CAD build for the part. Positions are in the model's coordinates, mm. Round coordinates to 2 decimals unless told otherwise and drop trailing zeros. Answer as a JSON object with one key per item and string values. Group by question number.
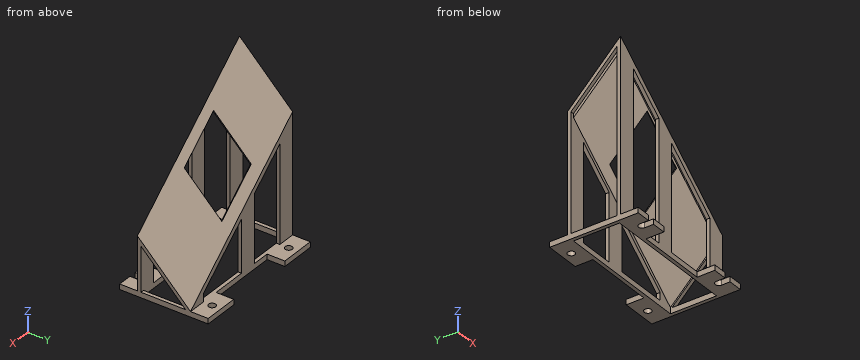
```python
from build123d import *

# Parameters (mm, degrees)
SKETCH_2_W           = 240
SKETCH_2_H           = 150
EXTRUDE_1_DEPTH      = 250
CUT_EXTRUDE_1_DEPTH  = 200
CUT_REVOLVE_1_ANGLE  = 37.4
SKETCH_13_W          = 80
SKETCH_13_H          = 100
CUT_EXTRUDE_2_DEPTH  = 295
SKETCH_14_W          = 160
SKETCH_14_H          = 150
CUT_EXTRUDE_3_DEPTH  = 295
SKETCH_16_W          = 80
SKETCH_16_H          = 28.16
CUT_EXTRUDE_4_DEPTH  = 295
SKETCH_22_W          = 80
SKETCH_22_H          = 9.999058643
CUT_EXTRUDE_5_DEPTH  = 120
SKETCH_23_W          = 80
SKETCH_23_H          = 9.99833939
CUT_EXTRUDE_6_DEPTH  = 142
SKETCH_24_W          = 80
SKETCH_24_H          = 11.98
CUT_EXTRUDE_7_DEPTH  = 142
SKETCH_25_W          = 20
SKETCH_25_H          = 3
EXTRUDE_2_DEPTH      = 10
SKETCH_26_W          = 20
SKETCH_26_H          = 3
EXTRUDE_3_DEPTH      = 10
SKETCH_27_W          = 20
SKETCH_27_H          = 3
EXTRUDE_4_DEPTH      = 10
SKETCH_28_W          = 20
SKETCH_28_H          = 3
EXTRUDE_5_DEPTH      = 10
SKETCH_29_R          = 1.997024656
CUT_EXTRUDE_8_DEPTH  = 10
SKETCH_30_R          = 1.996157305
CUT_EXTRUDE_9_DEPTH  = 10
CUT_EXTRUDE_10_DEPTH = 10
CUT_EXTRUDE_11_DEPTH = 10
SKETCH_34_W          = 76
SKETCH_34_H          = 26.002601967
CUT_EXTRUDE_14_DEPTH = 2
CUT_EXTRUDE_15_DEPTH = 2
CUT_EXTRUDE_17_DEPTH = 2
CUT_EXTRUDE_18_DEPTH = 2
CUT_EXTRUDE_20_DEPTH = 2
CUT_EXTRUDE_22_DEPTH = 2


with BuildPart() as part:
    # 草图2 → 凸台-拉伸1 (new body)
    with BuildSketch(Plane.XY):
        Rectangle(SKETCH_2_W, SKETCH_2_H)
    extrude(amount=EXTRUDE_1_DEPTH)

    # 草图9 → 切除-拉伸1 (cut)
    with BuildSketch(Plane(origin=(0, 75, 0), x_dir=(1, 0, 0), z_dir=(0, 1, 0))):
        Polygon((120, -250), (-120, -250), (208.236072982, 25.422767778), align=None)
    extrude(amount=-CUT_EXTRUDE_1_DEPTH, mode=Mode.SUBTRACT)

    # 草图10 → 切除-旋转1 (revolve, cut)
    with BuildSketch(Plane(origin=(73.519859787, 0, 87.617557028), x_dir=(0.7660444431189816, 0, -0.6427876096865353), z_dir=(0.6427876096865353, 0, 0.7660444431189817))):
        Polygon((60.675513844, -75), (-252.622235596, -75), (-252.622235596, 287.743692907), (60.675513844, 234.486341656), align=None)
    revolve(axis=Axis((120, -75, 48.616088517), (-0.7660444431189815, 0, 0.6427876096865353)), revolution_arc=CUT_REVOLVE_1_ANGLE, mode=Mode.SUBTRACT)

    # 草图13 → 切除-拉伸2 (cut)
    with BuildSketch(Plane(origin=(0, 0, 0), x_dir=(-1, 0, 0), z_dir=(0, 0, -1))):
        with Locations((80, -25)):
            Rectangle(SKETCH_13_W, SKETCH_13_H)
    extrude(amount=-CUT_EXTRUDE_2_DEPTH, mode=Mode.SUBTRACT)

    # 草图14 → 切除-拉伸3 (cut)
    with BuildSketch(Plane(origin=(0, 0, 0), x_dir=(-1, 0, 0), z_dir=(0, 0, -1))):
        with Locations((-40, 0)):
            Rectangle(SKETCH_14_W, SKETCH_14_H)
    extrude(amount=-CUT_EXTRUDE_3_DEPTH, mode=Mode.SUBTRACT)

    # 草图16 → 切除-拉伸4 (cut)
    with BuildSketch(Plane(origin=(0, 75, 0), x_dir=(1, 0, 0), z_dir=(0, 1, 0))):
        with Locations((-80, -14.08)):
            Rectangle(SKETCH_16_W, SKETCH_16_H)
    extrude(amount=-CUT_EXTRUDE_4_DEPTH, mode=Mode.SUBTRACT)

    # 草图22 → 切除-拉伸5 (cut)
    with BuildSketch(Plane(origin=(0, 0, 28.16), x_dir=(-1, 0, 0), z_dir=(0, 0, -1))):
        with Locations((80, 70.000470678)):
            Rectangle(SKETCH_22_W, SKETCH_22_H)
    extrude(amount=-CUT_EXTRUDE_5_DEPTH, mode=Mode.SUBTRACT)

    # 草图23 → 切除-拉伸6 (cut)
    with BuildSketch(Plane(origin=(0, 0, 28.16), x_dir=(-1, 0, 0), z_dir=(0, 0, -1))):
        with Locations((80, 29.999169695)):
            Rectangle(SKETCH_23_W, SKETCH_23_H)
    extrude(amount=-CUT_EXTRUDE_6_DEPTH, mode=Mode.SUBTRACT)

    # 草图24 → 切除-拉伸7 (cut)
    with BuildSketch(Plane(origin=(0, 65.000941357, 0), x_dir=(1, 0, 0), z_dir=(0, 1, 0))):
        with Locations((-80, -34.15)):
            Rectangle(SKETCH_24_W, SKETCH_24_H)
    extrude(amount=-CUT_EXTRUDE_7_DEPTH, mode=Mode.SUBTRACT)

    # 草图25 → 凸台-拉伸2 (add)
    with BuildSketch(Plane(origin=(0, 65.000941357, 0), x_dir=(1, 0, 0), z_dir=(0, 1, 0))):
        with Locations((-50, -41.64)):
            Rectangle(SKETCH_25_W, SKETCH_25_H)
    extrude(amount=EXTRUDE_2_DEPTH)

    # 草图26 → 凸台-拉伸3 (add)
    with BuildSketch(Plane(origin=(0, 65.000941357, 0), x_dir=(1, 0, 0), z_dir=(0, 1, 0))):
        with Locations((-110, -41.64)):
            Rectangle(SKETCH_26_W, SKETCH_26_H)
    extrude(amount=EXTRUDE_3_DEPTH)

    # 草图27 → 凸台-拉伸4 (add)
    with BuildSketch(Plane.XZ.offset(-34.99833939)):
        with Locations((-50, 41.64)):
            Rectangle(SKETCH_27_W, SKETCH_27_H)
    extrude(amount=EXTRUDE_4_DEPTH)

    # 草图28 → 凸台-拉伸5 (add)
    with BuildSketch(Plane.XZ.offset(-34.99833939)):
        with Locations((-110, 41.64)):
            Rectangle(SKETCH_28_W, SKETCH_28_H)
    extrude(amount=EXTRUDE_5_DEPTH)

    # 草图29 → 切除-拉伸8 (cut)
    with BuildSketch(Plane.XY.offset(43.14)):
        with Locations((-110, 69.998446832)):
            Circle(SKETCH_29_R)
    extrude(amount=-CUT_EXTRUDE_8_DEPTH, mode=Mode.SUBTRACT)

    # 草图30 → 切除-拉伸9 (cut)
    with BuildSketch(Plane.XY.offset(43.14)):
        with Locations((-50, 70.000941357)):
            Circle(SKETCH_30_R)
    extrude(amount=-CUT_EXTRUDE_9_DEPTH, mode=Mode.SUBTRACT)

    # 草图31 → 切除-拉伸10 (cut)
    with BuildSketch(Plane(origin=(0, 0, 40.14), x_dir=(-1, 0, 0), z_dir=(0, 0, -1))):
        with BuildLine():
            ThreePointArc((52, 29.962991919), (50, 31.962991919), (48, 29.962991919))
            Line((48, 29.962991919), (50, 29.962991919))
            Line((50, 29.962991919), (52, 29.962991919))
        make_face()
        with BuildLine():
            Line((48, 29.962991919), (48, 24.99833939))
            Line((48, 24.99833939), (50, 24.99833939))
            Line((50, 24.99833939), (50, 27.962991919))
            ThreePointArc((50, 27.962991919), (48.585786438, 28.548778357), (48, 29.962991919))
        make_face()
        with BuildLine():
            Line((50, 27.962991919), (50, 24.99833939))
            Line((50, 24.99833939), (52, 24.99833939))
            Line((52, 24.99833939), (52, 29.962991919))
            ThreePointArc((52, 29.962991919), (51.414213562, 28.548778357), (50, 27.962991919))
        make_face()
        with BuildLine():
            Line((50, 29.962991919), (48, 29.962991919))
            ThreePointArc((48, 29.962991919), (48.585786438, 28.548778357), (50, 27.962991919))
            Line((50, 27.962991919), (50, 29.962991919))
        make_face()
        with BuildLine():
            Line((50, 29.962991919), (50, 27.962991919))
            ThreePointArc((50, 27.962991919), (51.414213562, 28.548778357), (52, 29.962991919))
            Line((52, 29.962991919), (50, 29.962991919))
        make_face()
    extrude(amount=-CUT_EXTRUDE_10_DEPTH, mode=Mode.SUBTRACT)

    # 草图32 → 切除-拉伸11 (cut)
    with BuildSketch(Plane(origin=(0, 0, 40.14), x_dir=(-1, 0, 0), z_dir=(0, 0, -1))):
        with BuildLine():
            Line((112, 24.99833939), (112, 29.99833939))
            ThreePointArc((112, 29.99833939), (110, 31.99833939), (108, 29.99833939))
            Line((108, 29.99833939), (108, 24.99833939))
            Line((108, 24.99833939), (112, 24.99833939))
        make_face()
    extrude(amount=-CUT_EXTRUDE_11_DEPTH, mode=Mode.SUBTRACT)

    # 抽壳9: read off the stored shape, not the designer's step
    # 抽壳9: loft between two sections, ruled curve by curve
    shell_9_from = [
        Edge.make_line((-118, 36.99833939, 133.254360386), (-118, 36.99833939, 42.14)),
        Edge.make_line((-118, 36.99833939, 133.254360386), (-42, 36.99833939, 69.482788417)),
        Edge.make_line((-42, 36.99833939, 69.482788417), (-42, 36.99833939, 42.14)),
        Edge.make_line((-118, 36.99833939, 42.14), (-42, 36.99833939, 42.14)),
    ]
    shell_9_to = [
        Edge.make_line((-118, 63.000941357, 107.302223356), (-118, 63.000941357, 42.14)),
        Edge.make_line((-118, 63.000941357, 107.302223356), (-42, 63.000941357, 43.530651387)),
        Edge.make_line((-42, 63.000941357, 43.530651387), (-42, 63.000941357, 42.14)),
        Edge.make_line((-118, 63.000941357, 42.14), (-42, 63.000941357, 42.14)),
    ]
    shell_9 = Solid(Shell([*[Face.make_surface_from_curves(shell_9_from[k], shell_9_to[k]) for k in range(4)], Face(Wire(shell_9_from)), Face(Wire(shell_9_to))]))
    add(shell_9, mode=Mode.SUBTRACT)

    # 草图34 → 切除-拉伸14 (cut)
    with BuildSketch(Plane(origin=(0, 0, 40.14), x_dir=(-1, 0, 0), z_dir=(0, 0, -1))):
        with Locations((80, 49.999640374)):
            Rectangle(SKETCH_34_W, SKETCH_34_H)
    extrude(amount=-CUT_EXTRUDE_14_DEPTH, mode=Mode.SUBTRACT)

    # 草图35 → 切除-拉伸15 (cut)
    with BuildSketch(Plane.ZY.offset(120)):
        Polygon((43.14, 63.000941357), (109.441202222, 63.000941357), (135.393339252, 36.99833939), (43.14, 36.99833939), align=None)
    extrude(amount=-CUT_EXTRUDE_15_DEPTH, mode=Mode.SUBTRACT)

    # 草图37 → 切除-拉伸17 (cut)
    with BuildSketch(Plane(origin=(-40, 0, 0), x_dir=(0, 0, -1), z_dir=(1, 0, 0))):
        Polygon((-43.14, 36.99833939), (-68.265368758, 36.99833939), (-43.14, 62.172565402), align=None)
    extrude(amount=-CUT_EXTRUDE_17_DEPTH, mode=Mode.SUBTRACT)

    # 草图38 → 切除-拉伸18 (cut)
    with BuildSketch(Plane.XZ.offset(-34.99833939)):
        Polygon((-110, 43.14), (-110, 127.907923344), (-90, 111.12593072), (-90, 43.14), align=None)
        Polygon((-50, 43.14), (-50, 77.561945473), (-80, 102.734934409), (-80, 43.14), align=None)
    extrude(amount=-CUT_EXTRUDE_18_DEPTH, mode=Mode.SUBTRACT)

    # 草图39 → 切除-拉伸20 (cut)
    with BuildSketch(Plane(origin=(0, 65.000941357, 0), x_dir=(1, 0, 0), z_dir=(0, 1, 0))):
        Polygon((-110, -43.14), (-110, -97.963549373), (-90, -81.18155675), (-90, -43.14), align=None)
        Polygon((-50, -43.14), (-50, -47.617571503), (-80, -72.790560438), (-80, -43.14), align=None)
    extrude(amount=-CUT_EXTRUDE_20_DEPTH, mode=Mode.SUBTRACT)

    # 草图40 → 切除-拉伸22 (cut)
    with BuildSketch(Plane(origin=(23.136711502, 27.51974584, 27.573259053), x_dir=(0.8597946952762991, -0.3607260251766269, -0.3614274709191423), z_dir=(0.5106398750339969, 0.6073758397232878, 0.6085569055936306))):
        Polygon((-109.748917815, -9.755427356), (-136.477779275, -23.377760676), (-136.477779275, -53.377760676), (-109.748917815, -39.755427356), align=None)
    extrude(amount=-CUT_EXTRUDE_22_DEPTH, mode=Mode.SUBTRACT)


solid = part.part
```
Item 1: Drill centre lines: line 1 (Y direction, x = -50, z = 41.85); line 2 (X direction, y = 36, z = 65); line 3 (Y direction, x = -112.5, z = 91). Where is each one in solid material? Low to high. Write a range as [from, to].
Item 2: Flat gauge pins, fed straight in: pin 1 Ø3 at (x, y) = (-59, 58.5) entering from -Z; pin 2 Ø1.6 at (y, z) = (64.5, 65.5) entering from +X; pin 3 Ø1.6 at (y, z) = (64, 56) entering from +X. Where does each tip first touch, or does it go through?
Item 3: Cut at A-A, the plane z = 88.5. Give the number of separate pieces and of enclosed holes in the cut face, and give its area (3 significant figures).
Response values:
{
 "1": {"line 1": "[31.96, 37], [63, 68], [72, 75]", "line 2": "[-120, -110], [-90, -80], [-50, -40]", "line 3": "[35, 37], [63, 65]"},
 "2": {"pin 1": "z = 60.33", "pin 2": "x = -64.7", "pin 3": "x = -52.79"},
 "3": {"separate pieces": "5", "enclosed holes": "0", "area": "122 mm^2"}
}
